Read the model definition and answer for the solid it produces. Units are mm, in the model's axes. A direction names the side the tool comes from. Round coordinates to 2 decimals unless told otherwise and drop trailing zeros. Write each loop counter-clockwise with the first axis right and the second up, starting at its lowest first coordinate (ties: lowest second). Pieces come first, ordered by that corner, then holes.
from build123d import *

# Parameters (mm, degrees)
SKETCH_1_W      = 92.075
SKETCH_1_H      = 8
SKETCH_1_R      = 1.6
SKETCH_1_W_2    = 12.5
SKETCH_1_H_2    = 20
SKETCH_1_W_3    = 15
SKETCH_1_H_3    = 14.5
EXTRUDE_1_DEPTH = 5


with BuildPart() as part:
    # 草图1 → 凸台-拉伸1 (new body)
    # profile 1 of 7: a face of its own
    with BuildSketch(Plane.XY):
        with Locations((0, 28.5)):
            Rectangle(SKETCH_1_W, SKETCH_1_H)
        with Locations((41.9735, 28.92)):
            Circle(SKETCH_1_R, mode=Mode.SUBTRACT)
        with Locations((-41.9735, 28.92)):
            Circle(SKETCH_1_R, mode=Mode.SUBTRACT)
    # profile 2 of 7: a face of its own
    with BuildSketch(Plane.XY):
        with Locations((13.75, 0)):
            Rectangle(SKETCH_1_W_2, SKETCH_1_H_2)
    # profile 3 of 7: a face of its own
    with BuildSketch(Plane.XY):
        Rectangle(SKETCH_1_W_3, SKETCH_1_H_2)
    # profile 4 of 7: a face of its own
    with BuildSketch(Plane.XY):
        with Locations((-13.75, 0)):
            Rectangle(SKETCH_1_W_2, SKETCH_1_H_2)
    # profile 5 of 7: a face of its own
    with BuildSketch(Plane.XY):
        with Locations((0, 17.25)):
            Rectangle(SKETCH_1_W_3, SKETCH_1_H_3)
    # profile 6 of 7: a face of its own
    with BuildSketch(Plane.XY):
        with Locations((0, -28.5)):
            Rectangle(SKETCH_1_W, SKETCH_1_H)
        with Locations((-41.9735, -28.92)):
            Circle(SKETCH_1_R, mode=Mode.SUBTRACT)
        with Locations((41.9735, -28.92)):
            Circle(SKETCH_1_R, mode=Mode.SUBTRACT)
    # profile 7 of 7: a face of its own
    with BuildSketch(Plane.XY):
        with Locations((0, -17.25)):
            Rectangle(SKETCH_1_W_3, SKETCH_1_H_3)
    extrude(amount=EXTRUDE_1_DEPTH)


solid = part.part
Q1. Section B-B (y = 28.92) is taken. Determine the outline of the cut face in (x, z), then the cut area to 3 significant figures.
Verdict:
outline: (-46.04, 0) - (-43.57, 0) - (-43.57, 5) - (-46.04, 5) - close; (-40.37, 0) - (40.37, 0) - (40.37, 5) - (-40.37, 5) - close; (43.57, 0) - (46.04, 0) - (46.04, 5) - (43.57, 5) - close
area: 428 mm2
Q2. Section C-C (z = 3.05) is taken. Determine the outline of the cut face in (x, y), then the cut area to 3 significant figures.
Verdict:
outline: (-46.04, -32.5) - (46.04, -32.5) - (46.04, -24.5) - (7.5, -24.5) - (7.5, -10) - (20, -10) - (20, 10) - (7.5, 10) - (7.5, 24.5) - (46.04, 24.5) - (46.04, 32.5) - (-46.04, 32.5) - (-46.04, 24.5) - (-7.5, 24.5) - (-7.5, 10) - (-20, 10) - (-20, -10) - (-7.5, -10) - (-7.5, -24.5) - (-46.04, -24.5) - close; hole circle Ø3.2 at (-41.97, -28.92); hole circle Ø3.2 at (-41.97, 28.92); hole circle Ø3.2 at (41.97, -28.92); hole circle Ø3.2 at (41.97, 28.92)
area: 2,680 mm2
Q3. Straight lines are drawn through the part: probe 1 along Y at (x, z) = (-9, 3.15); probe 2 along Y at (x, z) = (32, 1.7); probe 3 along X at (y, z) = (-29, 2.55). For each, find the intervals that lie inside material, in ascending order.
Verdict:
probe 1: y = -32.5 to -24.5, -10 to 10, 24.5 to 32.5
probe 2: y = -32.5 to -24.5, 24.5 to 32.5
probe 3: x = -46.04 to -43.57, -40.38 to 40.38, 43.57 to 46.04
Q4. Flat-ended cylindrical pins translate along their axes: pin 1 Ø1 at (y, z) = (20.5, 4) entering from -X; pin 2 Ø3 at (y, z) = (4, 3) entering from +X; pin 3 Ø2 at (y, z) = (2, 2) entering from -X. Find the tip coordinate at first contact, or state that the pin passes through.
Verdict:
pin 1: stops at x = -7.5
pin 2: stops at x = 20
pin 3: stops at x = -20
Q5. Determine the mould class of faces 1 (the flat face through (-20, 0, 2)), 2 (the flat face through (-1, 32.5, 2)), 3 (the flat face through (-1, 0, 0)) for opening direction Y: pulls with the +Y half, pulls with the -Y half, needs draft (parallel to the pull), parting line crosses it, or undercut.
Verdict:
face 1: undercut
face 2: pulls with the +Y half
face 3: needs draft
Q6. Which of the six approach directions +Z, -Z, +X, -X, +Y, -Y give full straight-line access (tool end or side, diameter ignored) to faces 4 (the flat face through (-7.5, -17, 2)), 5 (the flat face through (14, -10, 2)), 6 (the cylindrical face through (40.7, 27.95, 2.46))?
Verdict:
face 4: +Z, -Z, -X
face 5: +Z, -Z, +X
face 6: +Z, -Z
Q7. Section D-D (x = 22) is taken. Determine the outline of the cut face in (y, z), then the cut area to 3 significant figures.
Verdict:
outline: (-32.5, 0) - (-24.5, 0) - (-24.5, 5) - (-32.5, 5) - close; (24.5, 0) - (32.5, 0) - (32.5, 5) - (24.5, 5) - close
area: 80.0 mm2
Q8. Section A-A (x = -8.5) is taken. Determine the outline of the cut face in (y, z), then the cut area to 3 significant figures.
Verdict:
outline: (-32.5, 0) - (-24.5, 0) - (-24.5, 5) - (-32.5, 5) - close; (-10, 0) - (10, 0) - (10, 5) - (-10, 5) - close; (24.5, 0) - (32.5, 0) - (32.5, 5) - (24.5, 5) - close
area: 180 mm2
